Part model, mm, in its own coordinate system. Face numbers are marked on the shaded views. A direction names the side the tool comes from. Round coordinates to 2 decimals unless told otherwise and drop trailing zeros. Loops run counter-clockwise (first coordinate to the right, second up) from the corner with the lowest first, then second, coordinate; pieces in that order, holes last. Notation, with made-up numbers: (-35.5, 64) - (-20.5, 64) arc R20 ccw to (-20.5, 90) - close; hole circle Ø11 at (-18.75, 76). An arc over 180 degrees is marked (long way). Put each result on its own line as item: value.
from build123d import *


with BuildPart() as part:
    # Sketch1 → Revolve2 (revolve)
    with BuildSketch(Plane.XY):
        with BuildLine():
            Line((45.639160326, 28.298601183), (95.74633283, 9.064259762))
            ThreePointArc((95.74633283, 9.064259762), (102.791629792, 7.077280519), (110.081050812, 6.407476822))
            Line((110.081050812, 6.407476822), (127.851823553, 6.407476822))
            ThreePointArc((127.851823553, 6.407476822), (139.546691742, 8.155286583), (150.219539692, 13.24597392))
            Line((150.219539692, 13.24597392), (246.802204076, 78.391803626))
            Line((246.802204076, 78.391803626), (246.802204076, 83.391803626))
            Line((246.802204076, 83.391803626), (43.876590917, 41.163939374))
            ThreePointArc((43.876590917, 41.163939374), (34.757151884, 39.749500606), (25.540810641, 39.276362798))
            Line((25.540810641, 39.276362798), (-17.770606993, 39.276362798))
            Line((-17.770606993, 39.276362798), (-17.770606993, 34.276362798))
            Line((-17.770606993, 34.276362798), (13.386044867, 34.276362798))
            ThreePointArc((13.386044867, 34.276362798), (29.787242162, 32.769304479), (45.639160326, 28.298601183))
        make_face()
    revolve(axis=Axis((-9.079018431, -13.592523178, 0), (1, 0, 0)))


solid = part.part
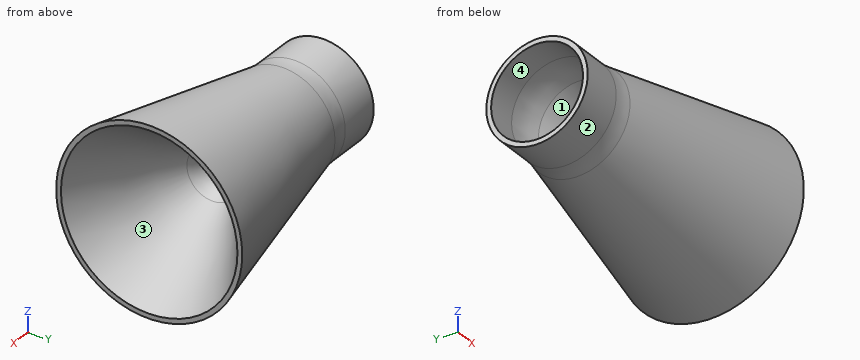
1. Band-saw the part on A-A (x = 184.5). List the corners of the cut face in (y, z).
A:
outline: circle Ø168.04 at (-13.59, 0); hole circle Ø99.92 at (-13.59, 0)
2. Pin check, flat tips, straight feed: P1, Ø2, axis at y = -58, z = -12, coming from the +X side; P2, Ø10, axis at x = 74, z = 19, coming from the +Y side; P3, Ø1.5, axis at y = -59, z = 77.5, coming from the +X side. Stop position of each tip, or through.
A:
P1: stops at x = 180.11
P2: stops at y = 46.21
P3: stops at x = 244.71
3. Band-saw the part on B-B (x = 83.5). List the corners of the cut face in (y, z).
A:
outline: circle Ø126 at (-13.59, 0); hole circle Ø54.72 at (-13.59, 0)
4. Two-plate mould, pull along Z, no slides. Class the marked faces 1 and 2: pulls with the +Z half, pulls with the -Z half, needs draft (parallel to the pull), parting line crosses it, or undercut.
A:
face 1: undercut
face 2: parting line crosses it
5. Probe line 1 along Y through (x, z) = (156, -3); line 2 along Z through (x, y) = (7, -39.5); line 3 along Y through (x, z) = (25, -35.5). List the from-to ranges inside material, lowest first. Write a range as [from, to].
A:
line 1: y = [-91.62, -44.18], [17, 64.44]
line 2: z = [-46.09, -40.25], [40.25, 46.09]
line 3: y = [-52.77, -44.57], [17.39, 25.58]
6. Tool access for the marked faces 3 and 4: list every direction of +Z, -Z, +X, -X, +Y, -Y with a clear straight run to the whole face (end or side of a thin tool).
A:
face 3: +X
face 4: -X
